```python
from build123d import *

# Parameters (mm, degrees)
ESBO_O1_R                   = 55
RESSALTO_EXTRUS_O1_DEPTH    = 115
ESBO_O2_R                   = 45
RESSALTO_EXTRUS_O2_DEPTH    = 60
ESBO_O3_R                   = 4.5
CORTE_EXTRUS_O1_DEPTH       = 6
FILETE1_R                   = 2.5
ESBO_O10_R                  = 4.5
CORTE_EXTRUS_O7_DEPTH       = 7.5
CORTE_EXTRUS_O8_REACH       = 168.752
CORTE_EXTRUS_O8_END_RADIUS  = 55
ESBO_O11_R                  = 8.5
CORTE_EXTRUS_O12_DEPTH      = 6.7
ESBO_O17_R                  = 4.5
CORTE_EXTRUS_O13_DEPTH      = 15
CORTE_EXTRUS_O14_DEPTH      = 15
CORTE_EXTRUS_O14_DEPTH_BACK = 15
ESBO_O18_R                  = 1.95
ESBO_O19_W                  = 50
ESBO_O19_H                  = 20
CORTE_EXTRUS_O15_DEPTH      = 53
CORTE_EXTRUS_O16_REACH      = 146.099
ESBO_O20_W                  = 13
ESBO_O20_H                  = 6.7
ESBO_O21_W                  = 10
ESBO_O21_H                  = 20
RESSALTO_EXTRUS_O4_DEPTH    = 30.9
CORTE_EXTRUS_O17_DEPTH      = 39.05
CORTE_EXTRUS_O17_DEPTH_BACK = 9.05
ESBO_O22_W                  = 5.8
ESBO_O22_H                  = 3.2
ESBO_O23_R                  = 1.6
CORTE_EXTRUS_O18_DEPTH      = 10
RESSALTO_EXTRUS_O5_START    = 10
ESBO_O24_R                  = 55
ESBO_O24_R_2                = 47.5
RESSALTO_EXTRUS_O5_DEPTH    = 10


with BuildPart() as part:
    # Esboço1 → Ressalto-extrusão1 (new body)
    with BuildSketch(Plane.XY):
        Circle(ESBO_O1_R)
    extrude(amount=RESSALTO_EXTRUS_O1_DEPTH)

    # Esboço2 → Ressalto-extrusão2 (add)
    with BuildSketch(Plane(origin=(0, 0, 0), x_dir=(1, 0, 0), z_dir=(0, 1, 0))):
        with Locations(Location((0, -67.5, 0), (0, 0, 90))):
            Circle(ESBO_O2_R)
    extrude(amount=RESSALTO_EXTRUS_O2_DEPTH)

    # Esboço3 → Corte-extrusão1 (cut)
    with BuildSketch(Plane(origin=(0, 0, 0), x_dir=(-1, 0, 0), z_dir=(0, 0, -1))):
        Circle(ESBO_O3_R)
    extrude(amount=-CORTE_EXTRUS_O1_DEPTH, mode=Mode.SUBTRACT)

    # Filete1
    filete1_edges = [part.edges().sort_by_distance(p)[0] for p in [
        (-55, 0, 115),
    ]]
    fillet(filete1_edges, radius=FILETE1_R - 0.0001)  # a hair under: the kernel refuses the full size

    # Esboço10 → Corte-extrusão7 (cut)
    with BuildSketch(Plane(origin=(0, 60, 0), x_dir=(1, 0, 0), z_dir=(0, 1, 0))):
        with Locations(Location((0, -67.5, 0), (0, 0, 270))):
            Circle(ESBO_O10_R)
    extrude(amount=-CORTE_EXTRUS_O7_DEPTH, mode=Mode.SUBTRACT)

    # Corte-extrusão8: up to this cylinder (the profile starts inside it)
    corte_extrus_o8_end = Plane(origin=(0, 0, 67.5), z_dir=(0, 0, -1)) * Cylinder(CORTE_EXTRUS_O8_END_RADIUS, 448.504, mode=Mode.PRIVATE)
    # Esboço11 → Corte-extrusão8 (cut, up to the surface)
    with BuildSketch(Plane(origin=(0, 52.5, 0), x_dir=(1, 0, 0), z_dir=(0, 1, 0)), mode=Mode.PRIVATE) as corte_extrus_o8_sk1:
        with Locations(Location((0, -67.5, 0), (0, 0, 270))):
            Circle(ESBO_O11_R)
    corte_extrus_o8_tool1 = extrude(corte_extrus_o8_sk1.sketch, amount=-CORTE_EXTRUS_O8_REACH, mode=Mode.PRIVATE) & corte_extrus_o8_end
    add(corte_extrus_o8_tool1.solids().sort_by_distance((0, 52.5, 67.5))[0], mode=Mode.SUBTRACT)

    # Esboço16 → Corte-extrusão12 (cut)
    with BuildSketch(Plane(origin=(0, 0, 6), x_dir=(-1, 0, 0), z_dir=(0, 0, -1))):
        with BuildLine():
            Line((-6.5, 3.073450829), (-6.5, -7.19))
            Line((-6.5, -7.19), (6.5, -7.19))
            Line((6.5, -7.19), (6.5, 3.073450829))
            ThreePointArc((6.5, 3.073450829), (0, 7.19), (-6.5, 3.073450829))
        make_face()
    extrude(amount=-CORTE_EXTRUS_O12_DEPTH, mode=Mode.SUBTRACT)

    # Esboço17 → Corte-extrusão13 (cut)
    with BuildSketch(Plane(origin=(0, 0, 12.7), x_dir=(-1, 0, 0), z_dir=(0, 0, -1))):
        Circle(ESBO_O17_R)
    extrude(amount=-CORTE_EXTRUS_O13_DEPTH, mode=Mode.SUBTRACT)

    # Esboço18 → Corte-extrusão14 (cut, two sides: drawn at the far end of the back side and taken through both)
    with BuildSketch(Plane(origin=(0, 0, 0), x_dir=(1, 0, 0), z_dir=(0, 1, 0)).offset(-CORTE_EXTRUS_O14_DEPTH_BACK)):
        with Locations(Location((0, -17.8, 0), (0, 0, 90))):
            Circle(ESBO_O18_R)
    extrude(amount=CORTE_EXTRUS_O14_DEPTH + CORTE_EXTRUS_O14_DEPTH_BACK, mode=Mode.SUBTRACT)

    # Esboço19 → Corte-extrusão15 (cut)
    with BuildSketch(Plane(origin=(0, -15, 0), x_dir=(1, 0, 0), z_dir=(0, 1, 0))):
        with Locations((0, -15)):
            Rectangle(ESBO_O19_W, ESBO_O19_H)
    extrude(amount=-CORTE_EXTRUS_O15_DEPTH, mode=Mode.SUBTRACT)

    # Esboço20 → Corte-extrusão16 (cut, up to next)
    with BuildSketch(Plane(origin=(0, -7.19, 0), x_dir=(1, 0, 0), z_dir=(0, 1, 0)), mode=Mode.PRIVATE) as corte_extrus_o16_sk1:
        with Locations((0, -9.35)):
            Rectangle(ESBO_O20_W, ESBO_O20_H)
    corte_extrus_o16_tool1 = extrude(corte_extrus_o16_sk1.sketch, amount=-CORTE_EXTRUS_O16_REACH, mode=Mode.PRIVATE) & part.part
    add(corte_extrus_o16_tool1.solids().sort_by_distance((0, -7.19, 9.35))[0], mode=Mode.SUBTRACT)

    # Esboço21 → Ressalto-extrusão4 (add)
    with BuildSketch(Plane.XZ.offset(15)):
        with Locations((20, 15)):
            Rectangle(ESBO_O21_W, ESBO_O21_H)
        with Locations((-20, 15)):
            Rectangle(ESBO_O21_W, ESBO_O21_H)
    extrude(amount=RESSALTO_EXTRUS_O4_DEPTH)

    # Esboço22 → Corte-extrusão17 (cut, two sides: drawn at the far end of the back side and taken through both)
    with BuildSketch(Plane.ZY.offset(-15).offset(-CORTE_EXTRUS_O17_DEPTH_BACK)):
        with Locations((15, -41.3)):
            Rectangle(ESBO_O22_W, ESBO_O22_H)
    extrude(amount=CORTE_EXTRUS_O17_DEPTH + CORTE_EXTRUS_O17_DEPTH_BACK, mode=Mode.SUBTRACT)

    # Esboço23 → Corte-extrusão18 (cut)
    with BuildSketch(Plane.XZ.offset(45.9)):
        with Locations(Location((21, 15, 0), (0, 0, 270))):
            Circle(ESBO_O23_R)
        with Locations(Location((-21, 15, 0), (0, 0, 270))):
            Circle(ESBO_O23_R)
    extrude(amount=-CORTE_EXTRUS_O18_DEPTH, mode=Mode.SUBTRACT)

    # Esboço24 → Ressalto-extrusão5 (add)
    with BuildSketch(Plane(origin=(0, 0, 0), x_dir=(-1, 0, 0), z_dir=(0, 0, -1)).offset(RESSALTO_EXTRUS_O5_START)):
        Circle(ESBO_O24_R)
        Circle(ESBO_O24_R_2, mode=Mode.SUBTRACT)
    extrude(amount=-RESSALTO_EXTRUS_O5_DEPTH)


solid = part.part
```
Could you check a few things on this model? Use its own coordinates, in mm. A direction names the side the tool comes from. Round coordinates to 2 decimals unless told otherwise and drop trailing zeros. Loops run counter-clockwise (first coordinate to the right, second up) from the corner with the lowest first, then second, coordinate; pieces in that order, holes last. Notation, with made-up numbers: (-25.75, 60.25) - (-20.75, 60.25) arc R4 cw to (-20.75, 67.25) - close; hole circle Ø4 at (9.5, -22). An arc over 180 degrees is marked (long way). Answer as CSV lines item,"result".
1. I want a section at D-D on z = 87.5. List the corners of the cut face in (x, y) for me.
Filled in:
outline,"(-40.31, 37.42) arc R55 ccw (long way) to (40.31, 37.42) - (40.31, 60) - (-40.31, 60) - close"
2. On a 3-axis mill with a long thin cutter (end or side, diameter ignored), from which of +Z, -Z, +X, -X, +Y, -Y can I reach the whole of each face in a straight line? I mean faces 4 (the face through (10.3, -46.37, -5.07)), 5 (the face through (24.05, -41, 15)), 6 (the face through (0, -6, 12.7)), 7 (the face through (-30.41, 48.77, 100.67)). Say none if no direction works.
Filled in:
face 4,"-Z"
face 5,"none"
face 6,"-Y"
face 7,"+Y"
3. Please list where these lines run through material, in increasing order: line 1 along Z through (x, y) = (0, -15.5); line 2 along Z through (x, y) = (4, -32.5); line 3 along Z through (x, y) = (0, 16). Write a range as [from, to].
Filled in:
line 1,"z = [0, 5], [25, 59], [76, 115]"
line 2,"z = [0, 5], [25, 60], [75, 115]"
line 3,"z = [0, 59], [76, 115]"
4. I want a section at C-C on z = 31. List the corners of the cut face in (x, y) for me, then the cut area to 3 significant figures.
Filled in:
outline,"(-26.32, 48.29) arc R55 ccw (long way) to (26.32, 48.29) - (26.32, 60) - (-26.32, 60) - close"
area,"9,880 mm^2"
5. For pin 1 Ø12 at (y, z) = (-12, 4.5) entering from -X; pin 2 Ø3.5 at (y, z) = (-42, 14) entering from +X; pin 3 Ø4 at (y, z) = (-15, 66) entering from -X, each with a flat end and sliding along its axis, tell me the tip position at first contact or that it passes through.
Filled in:
pin 1,"stops at x = -54.67"
pin 2,"stops at x = 37.48"
pin 3,"stops at x = -53.44"
6. I want a section at A-A on z = 65. List the corners of the cut face in (x, y) for me.
Filled in:
outline,"(-44.93, 31.72) arc R55 ccw to (-8.12, -54.4) - (-8.12, 52.5) - (-3.74, 52.5) - (-3.74, 60) - (-44.93, 60) - close; (3.74, 52.5) - (8.12, 52.5) - (8.12, -54.4) arc R55 ccw to (44.93, 31.72) - (44.93, 60) - (3.74, 60) - close"
7. We'd pull the mould along Z, two halves only. Please class faces 1 (the face through (45, -16, -10)), 2 (the face through (15, -30, 15)), 3 (the face through (-1, 1, 115)): +Z half, -Z half, draft (parallel to the pull), parting line (faces both ways), or undercut.
Filled in:
face 1,"-Z half"
face 2,"undercut"
face 3,"+Z half"
8. I want a section at B-B on y = 0. List the corners of the cut face in (x, z) for me.
Filled in:
outline,"(-55, -10) - (-47.5, -10) - (-47.5, 0) - (-4.5, 0) - (-4.5, 6) - (-6.5, 6) - (-6.5, 12.7) - (-4.5, 12.7) - (-4.5, 27.7) - (4.5, 27.7) - (4.5, 12.7) - (6.5, 12.7) - (6.5, 6) - (4.5, 6) - (4.5, 0) - (47.5, 0) - (47.5, -10) - (55, -10) - (55, 112.5) arc R2.5 ccw to (52.5, 115) - (-52.5, 115) arc R2.5 ccw to (-55, 112.5) - close; hole circle Ø17 at (0, 67.5)"
